Read the model definition and answer for the solid it produces. Units are mm, in the model's axes. A direction names the side the tool comes from. Coordinates: 2 decimals unless noted, no trailing zeros. Loops run counter-clockwise (first coordinate to the right, second up) from the corner with the lowest first, then second, coordinate; pieces in that order, holes last. Notation, with made-up numbers: (5, -16.75) - (50, -16.75) arc R17 cw to (50, 6.25) - close; hole circle Ø8 at (21.5, 86). An arc over 180 degrees is marked (long way). Use one line per item in the form item = value. Start each with the question number.
1) Each of these flat-tipped pins is pushed along its axis until it touches: P1, Ø6.5, axis at x = -23.5, y = -23.5, coming from the +Z side; P2, Ø6.5, axis at x = -15.5, y = -15.5, coming from the -Z side. Where does it stop, or does it pass through?
2) Which of the six approach directions +Z, -Z, +X, -X, +Y, -Y give full straight-line access (tool end or side, diameter ignored) to faces 1 (the face through (-15.76, -13.517, 29.154)), 2 (the face through (19.93, -25.52, 21.27))?
3) Consider line 1 (Y direction, x = -15.5, z = 27); line 2 (Y direction, x = -23.5, z = 22); line 3 (X direction, y = 15.5, z = 8.5). Determine where each line is inside the solid, lowest interval first.
4) A cutting plane is placed at B-B (y = 0). Give the vertices of the cut face in (x, z).
5) A cutting plane is placed at D-D (x = -23.5). Give the vertices of the cut face in (y, z).
6) A cutting plane is placed at C-C (y = -15.5). Give the vertices of the cut face in (x, z).
7) The mould has two halves that part along Y. Classify faces 3 (the face through (12.55, -18.2, 7.94)), 4 (the face through (30, 0, 20)), 5 (the face through (0, 30, 20)), 6 (the face through (-10.316, -7.91, 20.28)): released by +Y, released by -Y, zero draft, split by the parting line, or undercut.
8) A cutting plane is placed at A-A (x = -5). Give the vertices of the cut face in (y, z).
from build123d import *

# Parameters (mm, degrees)
F0_W      = 60
F0_H      = 60
F1_DEPTH  = 40
F2_R      = 2.75
F3_DEPTH  = 40
F4_R      = 2
F5_DEPTH  = 40
F6_R      = 13
F7_DEPTH  = 40
F8_R      = 1.5
F9_R      = 2.75
F10_DEPTH = 38
F11_R     = 4
F11_R_2   = 2
F12_DEPTH = 18
F13_R     = 1.9


with BuildPart() as f1:
    # F0 (on Top) → F1 (new body)
    with BuildSketch(Plane.XY):
        Rectangle(F0_W, F0_H)
    extrude(amount=F1_DEPTH)

    # F2 (on face) → F3 (cut, through all)
    with BuildSketch(Plane.XY.offset(40)):
        with Locations((-23.5, 23.5)):
            Circle(F2_R)
        with Locations((23.5, 23.5)):
            Circle(F2_R)
        with Locations((23.5, -23.5)):
            Circle(F2_R)
        with Locations((-23.5, -23.5)):
            Circle(F2_R)
    extrude(amount=-F3_DEPTH, mode=Mode.SUBTRACT)

    # F4 (on face) → F5 (cut, through all)
    with BuildSketch(Plane.XY.offset(40)):
        with Locations((-15.5, 15.5)):
            Circle(F4_R)
        with Locations((15.5, 15.5)):
            Circle(F4_R)
        with Locations((15.5, -15.5)):
            Circle(F4_R)
        with Locations((-15.5, -15.5)):
            Circle(F4_R)
    extrude(amount=-F5_DEPTH, mode=Mode.SUBTRACT)

    # F6 (on face) → F7 (cut, through all)
    with BuildSketch(Plane.XY.offset(40)):
        Circle(F6_R)
    extrude(amount=-F7_DEPTH, mode=Mode.SUBTRACT)

    # F8
    f8_edges = [f1.edges().sort_by_distance(p)[0] for p in [
        (30, -30, 20),
        (-30, -30, 20),
        (-30, 30, 20),
        (30, 30, 20),
    ]]
    fillet(f8_edges, radius=F8_R)

    # F9 (on face) → F10 (cut)
    with BuildSketch(Plane.XY.offset(40)):
        Polygon((21.132864, 19.4), (25.867136, 19.4), (28.234272, 23.5), (25.867136, 27.6), (21.132864, 27.6), (18.765728, 23.5), align=None)
        with Locations((23.5, 23.5)):
            Circle(F9_R, mode=Mode.SUBTRACT)
        Polygon((-25.867136, 19.4), (-21.132864, 19.4), (-18.765728, 23.5), (-21.132864, 27.6), (-25.867136, 27.6), (-28.234272, 23.5), align=None)
        Polygon((25.867136, -19.4), (21.132864, -19.4), (18.765728, -23.5), (21.132864, -27.6), (25.867136, -27.6), (28.234272, -23.5), align=None)
        Polygon((-21.132864, -19.4), (-25.867136, -19.4), (-28.234272, -23.5), (-25.867136, -27.6), (-21.132864, -27.6), (-18.765728, -23.5), align=None)
    extrude(amount=-F10_DEPTH, mode=Mode.SUBTRACT)

    # F11 (on face) → F12 (cut)
    with BuildSketch(Plane(origin=(0, 0, 0), x_dir=(1, 0, 0), z_dir=(0, 0, -1))):
        with Locations((15.5, 15.5)):
            Circle(F11_R)
        with Locations((15.5, 15.5)):
            Circle(F11_R_2, mode=Mode.SUBTRACT)
        with Locations((-15.5, 15.5)):
            Circle(F11_R)
        with Locations((-15.5, -15.5)):
            Circle(F11_R)
        with Locations((15.5, -15.5)):
            Circle(F11_R)
    extrude(amount=-F12_DEPTH, mode=Mode.SUBTRACT)

    # F13
    f13_edges = [f1.edges().sort_by_distance(p)[0] for p in [
        (11.5, 15.5, 18),
        (-19.5, 15.5, 18),
        (11.5, -15.5, 18),
        (-19.5, -15.5, 18),
    ]]
    fillet(f13_edges, radius=F13_R)


solid = f1.part
Found:
q1.P1 = 2
q1.P2 = 17.61
q2.face_1 = +Z, -Z
q2.face_2 = +Z
q3.line_1 = -30 to -17.5, -13.5 to 13.5, 17.5 to 30
q3.line_2 = -30 to -27.6, -19.4 to 19.4, 27.6 to 30
q3.line_3 = -30 to -19.5, -11.5 to 11.5, 19.5 to 30
q4.outline = (-30, 0) - (-13, 0) - (-13, 40) - (-30, 40) - close; (13, 0) - (30, 0) - (30, 40) - (13, 40) - close
q5.outline = (-30, 0) - (-26.25, 0) - (-26.25, 2) - (-27.6, 2) - (-27.6, 40) - (-30, 40) - close; (-20.75, 0) - (20.75, 0) - (20.75, 2) - (19.4, 2) - (19.4, 40) - (-19.4, 40) - (-19.4, 2) - (-20.75, 2) - close; (26.25, 0) - (30, 0) - (30, 40) - (27.6, 40) - (27.6, 2) - (26.25, 2) - close
q6.outline = (-30, 0) - (-19.5, 0) - (-19.5, 16.1) arc R1.9 cw to (-17.6, 18) - (-17.5, 18) - (-17.5, 40) - (-30, 40) - close; (-13.5, 18) - (-13.4, 18) arc R1.9 cw to (-11.5, 16.1) - (-11.5, 0) - (11.5, 0) - (11.5, 16.1) arc R1.9 cw to (13.4, 18) - (13.5, 18) - (13.5, 40) - (-13.5, 40) - close; (17.5, 18) - (17.6, 18) arc R1.9 cw to (19.5, 16.1) - (19.5, 0) - (30, 0) - (30, 40) - (17.5, 40) - close
q7.face_3 = undercut
q7.face_4 = zero draft
q7.face_5 = released by +Y
q7.face_6 = undercut
q8.outline = (-30, 0) - (-12, 0) - (-12, 40) - (-30, 40) - close; (12, 0) - (30, 0) - (30, 40) - (12, 40) - close
